Input: dimensioned drawing with shaded views. Units: mm. Origin: part minimum x, y, z. A direction names the side the tool comes from. Give positions to 0.01 mm unless a question says otherwise; leave off trailing zeros. Loops run counter-clockwise (first coordinate to the right, second up) from the corner with the lowest first, then second, coordinate; pieces in that order, holes last. Notation, with made-up numbers: (-30, 36.5) -> (2, 36.5) arc R24 cw to (2, 53.5) -> close; hole circle Ø7 at (68, 21). An arc over 180 degrees is marked (long way). Answer in a Markdown table with one row per item. Add a question column.
1) Access query for the marked faces 1 and 2. Directions: +Z, -Z, +X, -X, +Y, -Y. A direction counts if a zero-diameter tool reaches every point of the face in a straight line with its end or side. Return the directions, or none.
2) Line query: line 1 (Y direction, x = 12, z = 3.7); line 2 (Z direction, x = 13.5, y = 1); line 3 (Y direction, x = 5, z = 4.75). Output: solid intervals per line, ascending. Write a range as from..to.
3) Section query C-C (z = 4). Return the cut outline in (x, y).
4) Section query D-D (x = 4.75). Return the cut outline in (y, z), plus the area to 3 significant figures.
5) Section query B-B (y = 11). Return the cut outline in (x, z).
6) Section query A-A (x = 12). Return the cut outline in (y, z).
7) First-contact query: P1, Ø4, axis at x = 8, y = 1.5, coming from the +Z side; P2, Ø2, axis at x = 12.5, z = 3.5, coming from the -Y side. Flat tips, straight axial feed; report the tip coordinate or a pass-through.
8) Draft query along Y for the marked faces 3, 4 and 5. Return one class per face: +Y half, -Y half, draft (parallel to the pull), parting line (faces both ways), or undercut.
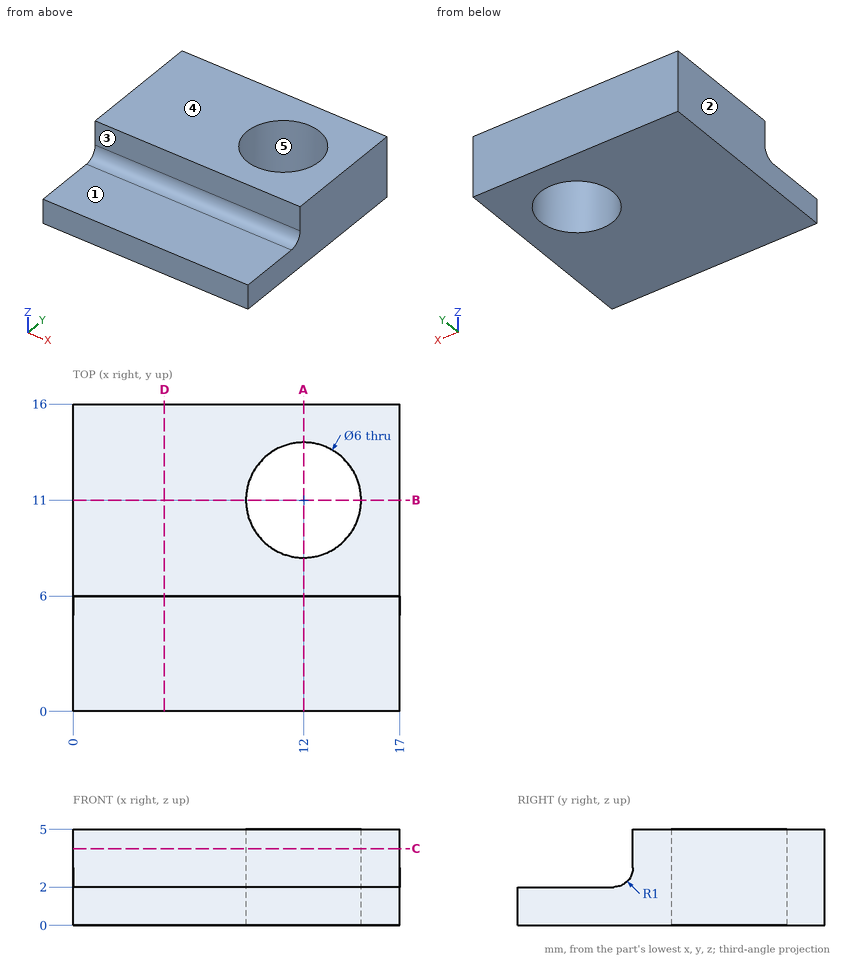
Evaluation:
| question | item | result |
|---|---|---|
| 1 | face 1 | +Z, +X, -X, -Y |
| 1 | face 2 | +Z, -Z, -X, +Y, -Y |
| 2 | line 1 | 6..8, 14..16 |
| 2 | line 2 | 0..2 |
| 2 | line 3 | 6..16 |
| 3 | outline | (0, 6) -> (17, 6) -> (17, 16) -> (0, 16) -> close; hole circle Ø6 at (12, 11) |
| 4 | outline | (0, 0) -> (16, 0) -> (16, 5) -> (6, 5) -> (6, 3) arc R1 cw to (5, 2) -> (0, 2) -> close |
| 4 | area | 62.2 mm² |
| 5 | outline | (0, 0) -> (9, 0) -> (9, 5) -> (0, 5) -> close; (15, 0) -> (17, 0) -> (17, 5) -> (15, 5) -> close |
| 6 | outline | (0, 0) -> (8, 0) -> (8, 5) -> (6, 5) -> (6, 3) arc R1 cw to (5, 2) -> (0, 2) -> close; (14, 0) -> (16, 0) -> (16, 5) -> (14, 5) -> close |
| 7 | P1 | z = 2 |
| 7 | P2 | y = 5.87 |
| 8 | face 3 | -Y half |
| 8 | face 4 | draft |
| 8 | face 5 | undercut |
